```python
from build123d import *

# Parameters (mm, degrees)
SKETCH_1_R                = 1.25
EXTRUDE_1_DEPTH           = 1.5
SKETCH_2_W                = 12
SKETCH_2_H                = 12
EXTRUDE_2_DEPTH           = 9.5
CUT_EXTRUDE_START         = 3.7
SKETCH_3_OUTSIDE_W        = 28.07
SKETCH_3_OUTSIDE_H        = 28.07
SKETCH_3_OUTSIDE_W_2      = 10.8
SKETCH_3_OUTSIDE_H_2      = 10.8
CUT_EXTRUDE_1_DEPTH       = 1.5
SKETCH_4_R                = 1.15
SKETCH_4_R_2              = 0.6
EXTRUDE_3_DEPTH           = 6.5
SKETCH_5_R                = 1.15
SKETCH_5_R_2              = 0.6
EXTRUDE_4_DEPTH           = 3
EXTRUDE_4_DRAFT           = 6
EXTRUDE_4_PROFILE_2_DEPTH = 3
EXTRUDE_4_PROFILE_2_DRAFT = 6
EXTRUDE_START             = -1.7
EXTRUDE_1_2_DEPTH         = 1.1
PATTERN_LINEAR_1_COUNT    = 4
PATTERN_LINEAR_1_PITCH    = 2.6
EXTRUDE_5_DEPTH           = 5
EXTRUDE_5_DEPTH_BACK      = 3
SKETCH_7_R                = 0.6


with BuildPart() as part:
    # Эскиз1 → Extrude 1 (new body)
    with BuildSketch(Plane(origin=(0, 0, 0), x_dir=(1, 0, 0), z_dir=(0, 1, 0))):
        with BuildLine():
            Line((2, 0), (18, 0))
            ThreePointArc((18, 0), (19.414213562, 0.585786438), (20, 2))
            Line((20, 2), (20, 18))
            ThreePointArc((20, 18), (19.414213562, 19.414213562), (18, 20))
            Line((18, 20), (2, 20))
            ThreePointArc((2, 20), (0.585786438, 19.414213562), (0, 18))
            Line((0, 18), (0, 2))
            ThreePointArc((0, 2), (0.585786438, 0.585786438), (2, 0))
        make_face()
        with Locations(Location((2.5, 2.5, 0), (0, 0, 270))):
            Circle(SKETCH_1_R, mode=Mode.SUBTRACT)
        with Locations(Location((17.5, 2.5, 0), (0, 0, 270))):
            Circle(SKETCH_1_R, mode=Mode.SUBTRACT)
    extrude(amount=EXTRUDE_1_DEPTH)

    # Эскиз2 → Бобышка-Вытянуть2 (add)
    with BuildSketch(Plane(origin=(0, 1.5, 0), x_dir=(1, 0, 0), z_dir=(0, 1, 0))):
        with Locations((10, 14)):
            Rectangle(SKETCH_2_W, SKETCH_2_H)
    extrude(amount=EXTRUDE_2_DEPTH)

    # Эскиз3 outside → Вырез-Вытянуть1 (cut)
    with BuildSketch(Plane(origin=(0, 1.5, 0), x_dir=(1, 0, 0), z_dir=(0, 1, 0)).offset(CUT_EXTRUDE_START)):
        with Locations((10, 10)):
            Rectangle(SKETCH_3_OUTSIDE_W, SKETCH_3_OUTSIDE_H)
        with Locations((10, 14)):
            Rectangle(SKETCH_3_OUTSIDE_W_2, SKETCH_3_OUTSIDE_H_2, mode=Mode.SUBTRACT)
    extrude(amount=CUT_EXTRUDE_1_DEPTH, mode=Mode.SUBTRACT)

    # Эскиз4 → Бобышка-Вытянуть3 (add)
    # profile 1 of 2: a face of its own
    with BuildSketch(Plane(origin=(0, 0, -20), x_dir=(-1, 0, 0), z_dir=(0, 0, -1))):
        with Locations(Location((-12.5, 9.85, 0), (0, 0, 90))):
            Circle(SKETCH_4_R)
        with Locations((-12.5, 9.85)):
            Circle(SKETCH_4_R_2, mode=Mode.SUBTRACT)
    # profile 2 of 2: a face of its own
    with BuildSketch(Plane(origin=(0, 0, -20), x_dir=(-1, 0, 0), z_dir=(0, 0, -1))):
        with Locations(Location((-7.5, 2.65, 0), (0, 0, 180))):
            Circle(SKETCH_4_R)
        with Locations((-7.5, 2.65)):
            Circle(SKETCH_4_R_2, mode=Mode.SUBTRACT)
    extrude(amount=EXTRUDE_3_DEPTH)


with BuildPart() as extrude_4_tool:
    # Эскиз5 → Бобышка-Вытянуть4 (with draft: the straight prism first)
    with BuildSketch(Plane(origin=(0, 0, -26.5), x_dir=(-1, 0, 0), z_dir=(0, 0, -1))):
        with Locations(Location((-7.5, 2.65, 0), (0, 0, 180))):
            Circle(SKETCH_5_R)
        with Locations((-7.5, 2.65)):
            Circle(SKETCH_5_R_2, mode=Mode.SUBTRACT)
    extrude(amount=-EXTRUDE_4_DEPTH)
    # Бобышка-Вытянуть4: the draft: its side faces are tilted about the plane it starts from
    extrude_4_sides = [extrude_4_tool.faces().sort_by_distance(p)[0] for p in [
        (6.35, 2.65, -25),
        (8.1, 2.65, -25),
    ]]
    draft(extrude_4_sides, Plane(origin=(0, 0, -26.5), x_dir=(-1, 0, 0), z_dir=(0, 0, -1)), EXTRUDE_4_DRAFT)


with BuildPart() as part_1:
    add(part.part)

    # Бобышка-Вытянуть4: add extrude_4_tool
    add(extrude_4_tool.part)


with BuildPart() as extrude_4_profile_2_tool:
    # Эскиз5 → Бобышка-Вытянуть4 profile 2 (with draft: the straight prism first)
    with BuildSketch(Plane(origin=(0, 0, -26.5), x_dir=(-1, 0, 0), z_dir=(0, 0, -1))):
        with Locations(Location((-12.5, 9.85, 0), (0, 0, 90))):
            Circle(SKETCH_5_R)
        with Locations((-12.5, 9.85)):
            Circle(SKETCH_5_R_2, mode=Mode.SUBTRACT)
    extrude(amount=-EXTRUDE_4_PROFILE_2_DEPTH)
    # Бобышка-Вытянуть4 profile 2: the draft: its side faces are tilted about the plane it starts from
    extrude_4_profile_2_sides = [extrude_4_profile_2_tool.faces().sort_by_distance(p)[0] for p in [
        (12.5, 8.7, -25),
        (13.1, 9.85, -25),
    ]]
    draft(extrude_4_profile_2_sides, Plane(origin=(0, 0, -26.5), x_dir=(-1, 0, 0), z_dir=(0, 0, -1)), EXTRUDE_4_PROFILE_2_DRAFT)


with BuildPart() as part_2:
    add(part_1.part)

    # Бобышка-Вытянуть4 profile 2: add extrude_4_profile_2_tool
    add(extrude_4_profile_2_tool.part)

    # Эскиз6 → Extrude 1 2 (add)
    with BuildSketch(Plane(origin=(0, 0, -20), x_dir=(-1, 0, 0), z_dir=(0, 0, -1)).offset(EXTRUDE_START)):
        Polygon((-15.4, 5.95), (-16.5, 5.95), (-17.4, 1.5), (-19, 1.5), (-19, 1.8), (-17.645399941, 1.8), (-16.745399941, 6.25), (-15.4, 6.25), align=None)
        Polygon((-1, 1.5), (-2.6, 1.5), (-3.5, 5.95), (-4.6, 5.95), (-4.6, 6.25), (-3.254600059, 6.25), (-2.354600059, 1.8), (-1, 1.8), align=None)
    extrude_1_2 = extrude(amount=-EXTRUDE_1_2_DEPTH)

    # Линейный массив1: Extrude 1 2 ×4
    with Locations(*[(0, 0, i * PATTERN_LINEAR_1_PITCH) for i in range(1, PATTERN_LINEAR_1_COUNT)]):
        add(extrude_1_2)

    # Эскиз7 → Бобышка-Вытянуть5 (add, two sides: drawn at the far end of the back side and taken through both)
    with BuildSketch(Plane.XY.offset(-EXTRUDE_5_DEPTH_BACK)):
        with Locations((8.95, 2)):
            Circle(SKETCH_7_R)
        with Locations((11.3, 2)):
            Circle(SKETCH_7_R)
        with Locations((13.65, 2)):
            Circle(SKETCH_7_R)
    extrude(amount=EXTRUDE_5_DEPTH + EXTRUDE_5_DEPTH_BACK)


solid = part_2.part
```
Model file for the job. Use its own axes, mm. A direction names the side the tool comes from. Give positions to 0.01 mm unless a question says otherwise; leave off trailing zeros. Order: outer loops, then holes, each group sorted by start corner. A loop starts at its lowest first (then second) coordinate and runs counter-clockwise, first axis right, second up.
1) Saw through at C-C, the plane x = 5.25. Write the cut outline in (y, z).
2) Pin check, flat tips, straight feed: pin 1 (1.1 mm diameter, centred on x = 17, y = 4, fed in from -Z); pin 2 (2 mm diameter, centred on x = 4, y = 2, fed in from +Z); pin 3 (4.5 mm diameter, centred on y = 9.5, z = -17, fed in from +X); pin 4 (4 mm diameter, centred on x = 3.5, z = -23.5, fed in from +Y). Stop position of each tip, or through.
3) Wall check: probe 1 along X at (y, z) = (1.15, -2.5); probe 2 along Y at (x, z) = (7.5, -22.2); probe 3 along Y at (x, z) = (12.5, -21.6). Give the ranges that are in metal, low to high.
4) Mould opens along Y. For faces 1 (the flat face through (10, 0, -10)), 2 (the flat face through (4, 6.25, -15)), 3 (the cylindrical face through (0.57, 0.74, -0.6)) say: +Y half, -Y half, draft (parallel to the pull), parting line (faces both ways), or undercut.
5) Saw through at D-D, the plane z = -11. Write the cut outline in (x, y), then the cut area to 3 significant figures.
6) 3-axis set-ups, long thin cutter, end or side, ignore diameter. For faces 4 (the cylindrical face through (13.1, 9.88, -21.73)), 5 (the flat face through (10, 9, -8)), 6 (the flat face through (4, 6.25, -10)), 7 (the flat face through (9, 2, -3)): which of +Z, -Z, +X, -X, +Y, -Y reach the whole face in a straight line?
7) Saw through at B-B, the plane z = -2.5. Write the cut outline in (x, y), then the cut area to 3 significant figures.
8) Saw through at A-A, the plane z = -21. Write the cut outline in (x, y), then the cut area to 3 significant figures.
Computed:
1. outline: (0, -20) - (5.2, -20) - (5.2, -19.4) - (6.7, -19.4) - (6.7, -20) - (11, -20) - (11, -8) - (6.7, -8) - (6.7, -8.6) - (5.2, -8.6) - (5.2, -8) - (1.5, -8) - (1.5, 0) - (0, 0) - close
2. pin 1: stops at z = -18.3
2. pin 2: stops at z = 0
2. pin 3: stops at x = 16
2. pin 4: passes through
3. probe 1: x = 0 to 1.25, 3.75 to 16.25, 18.75 to 20
3. probe 2: y = 1.5 to 2.05, 3.25 to 3.8
3. probe 3: y = 8.7 to 9.25, 10.45 to 11
4. face 1: -Y half
4. face 2: undercut
4. face 3: draft
5. outline: (0, 0) - (20, 0) - (20, 1.5) - (16, 1.5) - (16, 5.2) - (15.4, 5.2) - (15.4, 6.7) - (16, 6.7) - (16, 11) - (4, 11) - (4, 6.7) - (4.6, 6.7) - (4.6, 5.2) - (4, 5.2) - (4, 1.5) - (0, 1.5) - close
5. area: 142 mm2
6. face 4: none
6. face 5: +Z, +X, -X, +Y
6. face 6: +Z, -Z, -X
6. face 7: +X, -X, +Y
7. outline: (0, 0) - (1.25, 0) - (1.25, 1.5) - (0, 1.5) - close; (3.75, 0) - (16.25, 0) - (16.25, 1.5) - (13.98, 1.5) arc R0.6 ccw (long way) to (13.32, 1.5) - (11.63, 1.5) arc R0.6 ccw (long way) to (10.97, 1.5) - (9.28, 1.5) arc R0.6 ccw (long way) to (8.62, 1.5) - (3.75, 1.5) - close; (18.75, 0) - (20, 0) - (20, 1.5) - (18.75, 1.5) - close
7. area: 25.8 mm2
8. outline: circle Ø2.3 at (7.5, 2.65); circle Ø2.3 at (12.5, 9.85); hole circle Ø1.2 at (7.5, 2.65); hole circle Ø1.2 at (12.5, 9.85)
8. area: 6.05 mm2
